Design review of the part built by this model. Coordinates are the model's own, in mm. Face numbers are marked on the shaded views. A direction names the side the tool comes from. Coordinates: 2 decimals unless noted, no trailing zeros. Loops run counter-clockwise (first coordinate to the right, second up) from the corner with the lowest first, then second, coordinate; pieces in that order, holes last. Notation, with made-up numbers: (-23, -20.5) -> (31, -20.5) arc R19 ccw to (31, -8.5) -> close; hole circle Ø10 at (5.25, 21). An arc over 180 degrees is marked (long way). One line per item, written item: value. Start each with the question number.
1. Draft analysis for pull direction X (two halves, no side actions). For the marked faces 3, 4, 5 and 6, state which applies: pulls with the +X half, pulls with the -X half, needs draft (parallel to the pull), parting line crosses it, or undercut.
2. Machinability: for the marked faces 1 and 2, which of the approach directions +Z, -Z, +X, -X, +Y, -Y give a long, thin tool a straight path to every point of the face, cutting with its end or side? Answer none if there is none.
3. Add section B-B on y = 0. Write out the cut boundary in (x, z), plus the area to 3 significant figures.
4. For probe 1 along Y at (x, z) = (13, 3.5); probe 2 along Y at (x, z) = (3, 2); probe 3 along X at (y, z) = (-4, 6.25), list the stretches that pass through material, from the lowest coordinate up.
5. Add section C-C on x = -23.5. Write out the cut boundary in (y, z), plus the area to 3 significant figures.
6. Add section A-A on z = 2. Write out the cut boundary in (x, y), plus the area to 3 significant figures.
7. Insertion check: pin 1 (18 mm diameter, centred on x = -22, y = -12.7, fed in from +Z). The pin has a flat end and moves straight along its axis. Give the tip position at first contact, or say it passes through.
```python
from build123d import *

# Parameters (mm, degrees)
F1_DEPTH = 6.35
F0_R     = 11.15
F2_DEPTH = 6.35
F3_R     = 5.08


with BuildPart() as f1:
    # F0 (on Top) → F1 (new body)
    with BuildSketch(Plane.XY):
        Polygon((43.994091, -25.4), (0, 50.8), (-43.994091, -25.4), align=None)
        with BuildLine():
            ThreePointArc((-3.478961, 14.806637), (-6.539575, 34.430861), (11.15, 25.4))
            ThreePointArc((11.15, 25.4), (9.030861, 18.860425), (3.478961, 14.806637))
            ThreePointArc((3.478961, 14.806637), (6.838188, 13.58598), (9.819816, 11.615115))
            Line((9.819816, 11.615115), (20.002501, 11.656133))
            Line((20.002501, 11.656133), (14.946682, 2.81716))
            ThreePointArc((14.946682, 2.81716), (15.143919, 1.414713), (15.209855, 0))
            ThreePointArc((15.209855, 0), (15.047122, -2.218966), (14.562405, -4.39045))
            ThreePointArc((14.562405, -4.39045), (26.548213, -2.521131), (33.147045, -12.7))
            ThreePointArc((33.147045, -12.7), (20.849038, -23.790743), (11.083444, -10.416187))
            ThreePointArc((11.083444, -10.416187), (8.34671, -12.715035), (5.149077, -14.311768))
            Line((5.149077, -14.311768), (0.093257, -23.150741))
            Line((0.093257, -23.150741), (-5.033608, -14.352786))
            ThreePointArc((-5.033608, -14.352786), (-8.295423, -12.748554), (-11.083444, -10.416187))
            ThreePointArc((-11.083444, -10.416187), (-10.906302, -11.551993), (-10.847045, -12.7))
            ThreePointArc((-10.847045, -12.7), (-32.175914, -17.251168), (-14.562405, -4.39045))
            ThreePointArc((-14.562405, -4.39045), (-15.184898, -0.870945), (-14.968893, 2.696653))
            Line((-14.968893, 2.696653), (-20.095758, 11.494607))
            Line((-20.095758, 11.494607), (-9.913073, 11.535626))
            ThreePointArc((-9.913073, 11.535626), (-6.89286, 13.558324), (-3.478961, 14.806637))
        make_face(mode=Mode.SUBTRACT)
    extrude(amount=F1_DEPTH)

    # F0 (on Top) → F2 (join)
    with BuildSketch(Plane.XY):
        with BuildLine():
            ThreePointArc((15.209855, 0), (15.143919, 1.414713), (14.946682, 2.81716))
            Line((14.946682, 2.81716), (5.149077, -14.311768))
            ThreePointArc((5.149077, -14.311768), (8.34671, -12.715035), (11.083444, -10.416187))
            ThreePointArc((11.083444, -10.416187), (12.340862, -7.125), (14.562405, -4.39045))
            ThreePointArc((14.562405, -4.39045), (15.047122, -2.218966), (15.209855, 0))
        make_face()
        with BuildLine():
            ThreePointArc((3.478961, 14.806637), (0, 14.25), (-3.478961, 14.806637))
            ThreePointArc((-3.478961, 14.806637), (-6.89286, 13.558324), (-9.913073, 11.535626))
            Line((-9.913073, 11.535626), (9.819816, 11.615115))
            ThreePointArc((9.819816, 11.615115), (6.838188, 13.58598), (3.478961, 14.806637))
        make_face()
        with BuildLine():
            Line((-5.033608, -14.352786), (-14.968893, 2.696653))
            ThreePointArc((-14.968893, 2.696653), (-15.184898, -0.870945), (-14.562405, -4.39045))
            ThreePointArc((-14.562405, -4.39045), (-12.340862, -7.125), (-11.083444, -10.416187))
            ThreePointArc((-11.083444, -10.416187), (-8.295423, -12.748554), (-5.033608, -14.352786))
        make_face()
        with BuildLine():
            Line((9.819816, 11.615115), (-9.913073, 11.535626))
            ThreePointArc((-9.913073, 11.535626), (-13.202648, 7.551805), (-14.968893, 2.696653))
            Line((-14.968893, 2.696653), (-5.033608, -14.352786))
            ThreePointArc((-5.033608, -14.352786), (0.061269, -15.209731), (5.149077, -14.311768))
            Line((5.149077, -14.311768), (14.946682, 2.81716))
            ThreePointArc((14.946682, 2.81716), (13.141379, 7.657926), (9.819816, 11.615115))
        make_face()
        Circle(F0_R, mode=Mode.SUBTRACT)
    extrude(amount=F2_DEPTH)

    # F3
    f3_edges = [f1.edges().sort_by_distance(p)[0] for p in [
        (0, 50.8, 3.175),
        (43.994091, -25.4, 3.175),
        (-43.994091, -25.4, 3.175),
    ]]
    fillet(f3_edges, radius=F3_R)


solid = f1.part
```
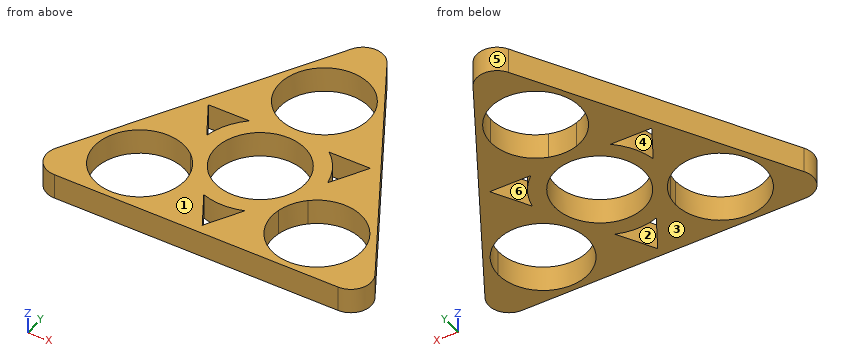
Worked answers:
1. face 3: needs draft
1. face 4: undercut
1. face 5: parting line crosses it
1. face 6: undercut
2. face 1: +Z, +X, -X, +Y, -Y
2. face 2: +Z, -Z
3. outline: (-29.33, 0) -> (-11.15, 0) -> (-11.15, 6.35) -> (-29.33, 6.35) -> close; (11.15, 0) -> (29.33, 0) -> (29.33, 6.35) -> (11.15, 6.35) -> close
3. area: 231 mm²
4. probe 1: y = -25.4 to -19.29, -6.11 to 7.9, 11.63 to 28.28
4. probe 2: y = -25.4 to -18.07, -14.91 to -10.74, 10.74 to 14.66, 36.14 to 44.74
4. probe 3: x = -31.64 to -28.97, -15.02 to -10.41, 10.41 to 15.02, 28.97 to 31.64
5. outline: (-25.4, 0) -> (-23.75, 0) -> (-23.75, 6.35) -> (-25.4, 6.35) -> close; (-1.65, 0) -> (10.1, 0) -> (10.1, 6.35) -> (-1.65, 6.35) -> close
5. area: 85.1 mm²
6. outline: (-39.59, -17.78) arc R5.08 ccw to (-35.2, -25.4) -> (35.2, -25.4) arc R5.08 ccw to (39.59, -17.78) -> (4.4, 43.18) arc R5.08 ccw to (-4.4, 43.18) -> close; hole (-20.1, 11.49) -> (-14.97, 2.7) arc R15.21 cw to (-9.91, 11.54) -> close; hole (-14.56, -4.39) arc R11.15 ccw (long way) to (-10.85, -12.7) arc R11.15 ccw to (-11.08, -10.42) arc R11.15 ccw to start; hole circle Ø22.3 at (0, 0); hole (-5.03, -14.35) -> (0.09, -23.15) -> (5.15, -14.31) arc R15.21 cw to start; hole (-3.48, 14.81) arc R11.15 ccw to (3.48, 14.81) arc R11.15 ccw to (11.15, 25.4) arc R11.15 ccw (long way) to start; hole (9.82, 11.62) arc R15.21 cw to (14.95, 2.82) -> (20, 11.66) -> close; hole (11.08, -10.42) arc R11.15 ccw (long way) to (14.56, -4.39) arc R11.15 ccw to start
6. area: 1,620 mm²
7. pin 1: passes through
